Design review of the part built by this model. Coordinates are the model's own, in mm. A direction names the side the tool comes from. Give positions to 0.01 mm unless a question says otherwise; leave off trailing zeros. Order: outer loops, then holes, each group sorted by start corner. A loop starts at its lowest first (then second) coordinate and runs counter-clockwise, first axis right, second up. Notation, with made-up numbers: (44.5, 40) - (50.5, 40) arc R9 cw to (50.5, 54) - close; hole circle Ø6 at (-4.5, 66). An arc over 180 degrees is marked (long way). Write each question's results on one line, items separated by ' | '. Start each with the question number.
Autodesk Inventor part; units mm, degrees
ref_plane "YZ Plane" through (0, 0, 0) normal (1, 0, 0) x (0, 1, 0)
ref_plane "XZ Plane" through (0, 0, 0) normal (0, 1, 0) x (-1, 0, 0)
ref_plane "XY Plane" through (0, 0, 0) normal (0, 0, 1) x (1, 0, 0)
sketch "Sketch1" plane through (0, 0, 0) normal (0, 1, 0) x (-1, 0, 0)
  line L0 (63.5, 50.8) -> (-63.5, 50.8)
  line L1 (-63.5, 50.8) -> (-63.5, -50.8)
  line L2 (-63.5, -50.8) -> (63.5, -50.8)
  line L3 (63.5, -50.8) -> (63.5, 50.8)
  line L4 (63.5, 50.8) -> (-63.5, -50.8) construction
  line L5 (-63.5, 50.8) -> (63.5, -50.8) construction
  point P0 (0, 0)
  dimension "d0" = 127
  dimension "d1" = 101.6
extrude "Extrusion1" add sketch "Sketch1" against normal blind 5.08
sketch "Sketch26" plane through (0, 0, 0) normal (0, 1, 0) x (1, 0, 0)
  line L0 (-21.5002, -11.0998) -> (36.4998, -11.0998) construction
  line L1 (36.4998, -11.0998) -> (36.4998, 11.9002) construction
  line L2 (36.4998, 11.9002) -> (-21.5002, 11.9002) construction
  line L3 (-21.5002, 11.9002) -> (-21.5002, -11.0998) construction
  line L4 (-63.5, -50.8) -> (63.5, -50.8) construction
  line L5 (63.5, -50.8) -> (-63.5, -50.8) construction
  circle A0 centre (-21.5002, -11.0998) radius 3
  circle A1 centre (-21.5002, 11.9002) radius 3
  circle A2 centre (36.4998, 11.9002) radius 3
  circle A3 centre (36.4998, -11.0998) radius 3
  line L6 (63.5, -50.8) -> (63.5, 50.8)
  line L7 (-21.5002, 0.4002) -> (36.4998, 0.4002) construction
  point P0 (0, 0)
  dimension "d173" = 58
  dimension "d174" = 23
  dimension "d175" = 39.7002
  dimension "d176" = 6
  dimension "d190" = 27.0002
  dimension "piZeroCenterLine" = 0.4002
extrude "Extrusion12" add sketch "Sketch26" along normal blind 2.54
sketch "Sketch27" plane through (0, -5.08, 0) normal (0, -1, 0) x (1, 0, 0)
  circle A0 centre (-21.5002, 11.0998) radius 3
  circle A1 centre (-21.5002, -11.9002) radius 3
  circle A2 centre (36.4998, -11.9002) radius 3
  circle A3 centre (36.4998, 11.0998) radius 3
  point P0 (0, 0)
hole "Hole17" at (-21.5002, -5.08, 11.0998) at (36.4998, -5.08, 11.0998) at (36.4998, -5.08, -11.9002) at (-21.5002, -5.08, -11.9002) direction (0, 1, 0) diameter 2.4384 end through all counterbore diameter 3.2639 counterbore depth 3.9878
sketch "Sketch28" plane through (0, 0, 0) normal (0, 1, 0) x (1, 0, 0)
  line L0 (63.5, -50.8) -> (-63.5, -50.8)
  line L1 (63.5, 50.8) -> (63.5, -50.8)
  line L2 (-63.5, -50.8) -> (63.5, -50.8)
  line L3 (63.5, -50.8) -> (63.5, 50.8)
  line L4 (63.5, 50.8) -> (-63.5, 50.8)
  line L5 (-63.5, 50.8) -> (-63.5, -50.8)
  line L6 (-62.23, -49.53) -> (62.23, -49.53)
  line L7 (62.23, -49.53) -> (62.23, 49.53)
  line L8 (62.23, 49.53) -> (-62.23, 49.53)
  line L9 (-62.23, 49.53) -> (-62.23, -49.53)
  line L10 (-62.23, -49.53) -> (62.23, 49.53) construction
  line L11 (62.23, -49.53) -> (-62.23, 49.53) construction
  point P0 (0, 0)
  dimension "d186" = 1.27
  dimension "d187" = 1.27
extrude "Extrusion13" add sketch "Sketch28" along normal blind 13.08
sketch "Sketch22" plane through (0, -5.08, 0) normal (0, -1, 0) x (1, 0, 0)
  point P0 (34.92, -17.42)
  point P1 (34.92, 17.42)
  point P2 (-34.92, 17.42)
  point P3 (-34.92, -17.42)
equation "\"d0\" = LargeCaseLength"
equation "\"d1\" = LargeCaseWidth"
equation "\"d2\" = CaseFloorThickness"
equation "\"d173\" = PiZeroMoutingHolesLength"
equation "\"d174\" = PiZeroMountingHolesWidth"
equation "\"d175\" = PiZeroHolesDistanceFromSideWall"
equation "\"d176\" = PiZeroHoleSupport"
equation "\"d190\" = PiZeroHolesDistanceFromBottomWall"
equation "\"d177\" = PiZeroWHoleHeight"
equation "\"d186\" = CaseWallThickness"
equation "\"d187\" = CaseWallThickness"
equation "\"d188\" = CaseHeight"
equation "\"PiZeroWLength\" = 65"
equation "\"PiZeroWWidth\" = 30"
equation "\"CaseLength\" = PiZeroWLength + 2 * EndOfCaseToStartOfPiZero"
equation "\"CaseWidth\" = PiZeroWWidth + 2 * EndOfCaseToStartOfPiZero"
equation "\"PiZeroWMountingHole\" = 2.75"
equation "\"CaseWallThickness\" = 1.27"
equation "\"CaseFloorThickness\" = 5.08"
equation "\"PiZeroMoutingHolesLength\" = 58"
equation "\"PiZeroMountingHolesWidth\" = 23"
equation "\"PiZeroHoleSupport\" = 6"
equation "\"PiZeroWHoleHeight\" = 2.54"
equation "\"PiRibbonCableWidth\" = 20"
equation "\"PiRibbonCableThickness\" = 5"
equation "\"HdmiCenter\" = 19"
equation "\"MiniUsbCenter\" = 41.4"
equation "\"PowerCenter\" = 54"
equation "\"HdmiWidth\" = 28"
equation "\"MiniUsbWidth\" = 18"
equation "\"PowerWidth\" = 20"
equation "\"EndOfCaseToStartOfPiZero\" = 7.5"
equation "\"EyepieceOutsideDiameter\" = 31.75"
equation "\"EyepieceWallThickness\" = 1.905"
equation "\"EyepieceInnerDiameter\" = EyepieceOutsideDiameter - 2 * EyepieceWallThickness"
equation "\"HeightOfConnectorHolesAboveBottom\" = 6"
equation "\"HdmiHightAboveBottom\" = 6"
equation "\"MiniUsbHeightAboveBottom\" = 5"
equation "\"PowerHeightAboveBottom\" = 5"
equation "\"PiRibbonCableHeightFromTp\" = 8.89"
equation "\"NutHeightPlusOffset\" = 1.8415"
equation "\"NutWidthPlusOffset\" = 5.0165"
equation "\"LargeCaseWidth\" = 101.6"
equation "\"LargeCaseLength\" = 127"
equation "\"CameraHoleLength\" = 12.58"
equation "\"CameraHoleWidth\" = 21"
properties part number "LargeCaseCaseBottomForPiZeroWV02" material "LCP Plastic"
Q1. Add section C-C (z = 30). Give the boundary of the cut face in (x, y).
Q2. Insertion check: pin 1 Ø3 at (x, z) = (-18.5, -39) entering from +Y; pin 2 Ø2 at (x, z) = (-21.5, 11.1) entering from +Y; pin 3 Ø6.5 at (x, z) = (-21.5, 10.5) entering from +Y; pin 4 Ø3 at (x, z) = (36.5, 11.1) entering from -Y. Each pin has a flat end and moves straight along its axis. Give the tip position at first contact, or say it passes through.
Q3. For line 1 (X direction, y = 9.5, z = 13); line 2 (Z direction, x = 45.5, y = 6.5); line 3 (Y direction, x = 24, z = -15), list the stretches that pass through material, from the lowest coordinate up. Write a range as [from, to].
Q4. Draft analysis for pull direction X (two halves, no side actions). For faces 4 (the flat face through (1, 4, -50.8)), 5 (the flat face through (62.23, 6, 1)), state which applies: pulls with the +X half, pulls with the -X half, needs draft (parallel to the pull), parting line crosses it, or undercut.
Q5. Add section A-A (y = 6.5). Give the boundary of the cut face in (x, z).
Q6. Add section B-B (x = 14). Give the boundary of the cut face in (y, z).
Q7. Machinability: for faces 1 (the flat face through (1, -5.08, 1)), 2 (the flat face through (1, 6, -49.53)), 3 (the cylindrical face through (37.12, -3.06, -13.41)), which of the approach directions +Z, -Z, +X, -X, +Y, -Y give a long, thin tool a straight path to every point of the face, cutting with its end or side? Answer none if there is none.
Verdict:
1) outline: (-63.5, -5.08) - (63.5, -5.08) - (63.5, 13.08) - (62.23, 13.08) - (62.23, 0) - (-62.23, 0) - (-62.23, 13.08) - (-63.5, 13.08) - close
2) pin 1: stops at y = 0 | pin 2: passes through | pin 3: stops at y = 2.54 | pin 4: stops at y = -1.09
3) line 1: x = [-63.5, -62.23], [62.23, 63.5] | line 2: z = [-50.8, -49.53], [49.53, 50.8] | line 3: y = [-5.08, 0]
4) face 4: needs draft | face 5: undercut
5) outline: (-63.5, -50.8) - (63.5, -50.8) - (63.5, 50.8) - (-63.5, 50.8) - close; hole (-62.23, -49.53) - (62.23, -49.53) - (62.23, 49.53) - (-62.23, 49.53) - close
6) outline: (-5.08, -50.8) - (13.08, -50.8) - (13.08, -49.53) - (0, -49.53) - (0, 49.53) - (13.08, 49.53) - (13.08, 50.8) - (-5.08, 50.8) - close
7) face 1: +Z, -Z, +X, -X, -Y | face 2: +Y | face 3: -Y
